from build123d import *

# Parameters (mm, degrees)
SKETCH1_W           = 132.7
SKETCH1_H           = 132.7
BOSS_EXTRUDE2_DEPTH = 6.35
SKETCH5_W           = 12.7
SKETCH5_H           = 16.35
CUT_EXTRUDE1_DEPTH  = 7.35
CIRPATTERN1_COUNT   = 2


with BuildPart() as part:
    # Sketch1 → Boss-Extrude2 (new body)
    with BuildSketch(Plane(origin=(0, 0, 0), x_dir=(1, 0, 0), z_dir=(0, 1, 0))):
        Rectangle(SKETCH1_W, SKETCH1_H)
    extrude(amount=BOSS_EXTRUDE2_DEPTH)

    # Sketch5 → Cut-Extrude1 (cut, through all)
    with BuildSketch(Plane(origin=(0, 6.35, 0), x_dir=(1, 0, 0), z_dir=(0, 1, 0))):
        with Locations((0, 58.175)):
            Rectangle(SKETCH5_W, SKETCH5_H)
    cut_extrude1 = extrude(amount=-CUT_EXTRUDE1_DEPTH, mode=Mode.SUBTRACT)

    # CirPattern1: Cut-Extrude1 ×2 about axis
    cirpattern1_axis = Axis((0, 0, 0), (0, 1, 0))
    for i in range(1, CIRPATTERN1_COUNT):
        add(cut_extrude1.rotate(cirpattern1_axis, i * 360 / CIRPATTERN1_COUNT), mode=Mode.SUBTRACT)


solid = part.part
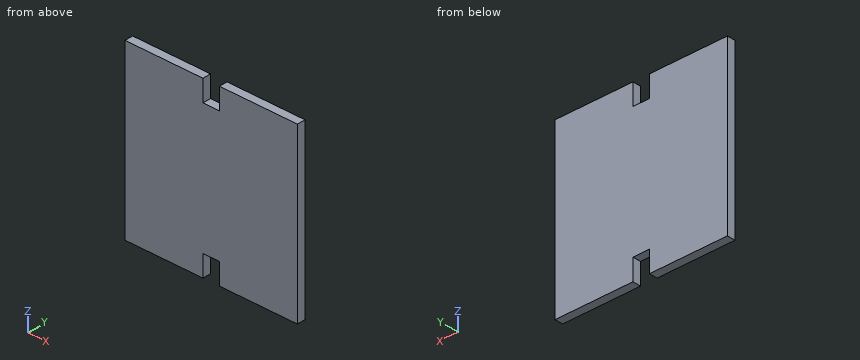
Can you work these out from the model? Positions are in its coordinate system, mm. Coordinates: 2 decimals unless noted, no trailing zeros. Loops run counter-clockwise (first coordinate to the right, second up) from the corner with the lowest first, then second, coordinate; pieces in that order, holes last. Notation, with made-up numbers: M 0.25,37.5 L 27.25,37.5 A12 cw 27.25,50.5 Z; hole C 24.25,-8.5 d3. An arc over 180 degrees is marked long. Answer as CSV lines item,"result". Start each with the question number.
1. For pin 1 Ø1.9 at (x, y) = (-1, 3) entering from +Z, with a flat end and sliding along its axis, tell me the tip position at first contact or that it passes through.
2. Suppose I cut it at B-B, the plane y = 3. List the corners of the cut face in (x, z) for me, plus the area to 3 significant figures.
3. Suppose I cut it at A-A, the plane z = 56. List the corners of the cut face in (x, y) for me, plus the area to 3 significant figures.
4. If I drill on probe 1 along X at (y, z) = (2.25, 57); probe 2 along Z at (x, y) = (4.5, 6.25), over which ranges is the centre line in solid material (lowest first)? Write a range as [from, to].
Output:
1,pin 1,"stops at z = 50"
2,outline,"M -66.35,-66.35 L -6.35,-66.35 L -6.35,-50 L 6.35,-50 L 6.35,-66.35 L 66.35,-66.35 L 66.35,66.35 L 6.35,66.35 L 6.35,50 L -6.35,50 L -6.35,66.35 L -66.35,66.35 Z"
2,area,"17,200 mm^2"
3,outline,"M -66.35,0 L -6.35,0 L -6.35,6.35 L -66.35,6.35 Z; M 6.35,0 L 66.35,0 L 66.35,6.35 L 6.35,6.35 Z"
3,area,"762 mm^2"
4,probe 1,"x = [-66.35, -6.35], [6.35, 66.35]"
4,probe 2,"z = [-50, 50]"
